Part model, mm, in its own coordinate system. A direction names the side the tool comes from. Coordinates: 2 decimals unless noted, no trailing zeros. Loops run counter-clockwise (first coordinate to the right, second up) from the corner with the lowest first, then second, coordinate; pieces in that order, holes last. Notation, with made-up numbers: (-23.5, 49.5) -> (-17.5, 49.5) arc R5 cw to (-17.5, 58.5) -> close; hole circle Ø7 at (-0.75, 52.5). An arc over 180 degrees is marked (long way). Use one line per item in the form item = value. Start each with the question number.
(1) 3-axis set-ups, long thin cutter, end or side, ignore diameter. For faces 5 (the flat face through (15.7, 2.5, -17.8)), 6 (the cylindrical face through (-14.635, 2.007, 6.999)), 7 (the cylindrical face through (11.5, 1, 6.9)): which of +Z, -Z, +X, -X, +Y, -Y reach the whole face in a straight line?
(2) Band-saw the part on B-B on x = 0. Count the separate pieces of the cut face and the enclosed holes in it, then the cut area to 3 significant figures.
(3) Band-saw the part on A-A on z = -5. Give the cut face in (x, y), then the cut area to 4 significant figures.
(4) Pin check, flat tips, straight feed: P1, Ø5, axis at x = 0, z = -5, coming from the -Y side; P2, Ø2, axis at x = 13, z = 6, coming from the +Y side; P3, Ø3, axis at y = 4.5, z = -34, coming from the +X side; P4, Ø0.5, axis at x = -13.5, y = 2, coming from the +Z side. Stop position of each tip, or through.
(5) Drill centre lines: L1, parallel to Z at x = 0, y = 0.3; L2, parallel to Z at x = -2.5, y = 0.6; L3, parallel to X at y = 0.35, z = -5. Where is each one in solid material? Low to high. Write a range as [from, to].
(6) Mould opens along X. For faces 1 (the flat face through (13, 2, 5.3)), 2 (the flat face through (11.92, 2, 6)), 3 (the cylindrical face through (-12.205, 2.007, 6.999)), 4 (the cylindrical face through (-17.08, 0.76, 12.4)) say: +X half, -X half, draft (parallel to the pull), parting line (faces both ways), or undercut.
```python
from build123d import *

# Parameters (mm, degrees)
SKETCH1_W               = 35.3
SKETCH1_H               = 26
BOSS_EXTRUDE1_DEPTH     = 1.5
SKETCH2_W               = 31.8
SKETCH2_H               = 1.5
BOSS_EXTRUDE2_DEPTH     = 3.8
CUT_EXTRUDE1_DEPTH      = 23.247752695
CUT_EXTRUDE1_DEPTH_BACK = 23.247752695
SKETCH3_R               = 2
CHAMFER1_SIZE           = 2
CHAMFER1_SIZE2          = 1
FILLET1_R               = 2
BOSS_EXTRUDE3_DEPTH     = 30
FILLET2_R               = 2
SKETCH6_W               = 3
SKETCH6_H               = 2
BOSS_EXTRUDE4_DEPTH     = 1
FILLET4_R               = 1
SKETCH7_W               = 1.743977538
SKETCH7_H               = 6.350659455
SKETCH7_W_2             = 2.282976844
SKETCH7_H_2             = 7.649157782
CUT_EXTRUDE2_DEPTH      = 37.494691395
CUT_EXTRUDE5_DEPTH      = 55.674605623
CUT_EXTRUDE5_DEPTH_BACK = 55.674605623
CUT_EXTRUDE6_DEPTH      = 47.63649323
CUT_EXTRUDE6_DEPTH_BACK = 47.63649323
CUT_EXTRUDE7_START      = -1.5
CUT_EXTRUDE7_DEPTH      = 1


with BuildPart() as part:
    # Sketch1 → Boss-Extrude1 (new body)
    with BuildSketch(Plane(origin=(0, 0, 0), x_dir=(1, 0, 0), z_dir=(0, 1, 0))):
        Rectangle(SKETCH1_W, SKETCH1_H)
    extrude(amount=BOSS_EXTRUDE1_DEPTH)

    # Sketch2 → Boss-Extrude2 (add)
    with BuildSketch(Plane(origin=(0, 1.5, 0), x_dir=(1, 0, 0), z_dir=(0, 1, 0))):
        with Locations((0, 12.25)):
            Rectangle(SKETCH2_W, SKETCH2_H)
    extrude(amount=BOSS_EXTRUDE2_DEPTH)

    # Sketch3 → Cut-Extrude1 (cut, two sides: drawn at the far end of the back side and taken through both)
    with BuildSketch(Plane(origin=(0, 1.5, 0), x_dir=(1, 0, 0), z_dir=(0, 1, 0)).offset(-CUT_EXTRUDE1_DEPTH_BACK)):
        with Locations(Location((0, 5, 0), (0, 0, 270))):
            Circle(SKETCH3_R)
    extrude(amount=CUT_EXTRUDE1_DEPTH + CUT_EXTRUDE1_DEPTH_BACK, mode=Mode.SUBTRACT)

    # Chamfer1
    chamfer1_edges = [part.edges().sort_by_distance(p)[0] for p in [
        (0, 1.5, -7),
    ]]
    chamfer1_side = [part.faces().sort_by_distance(p)[0] for p in [
        (0, 1.5, 0.754672273),
    ]]
    chamfer(chamfer1_edges, length=CHAMFER1_SIZE, length2=CHAMFER1_SIZE2, reference=chamfer1_side[0])

    # Fillet1
    fillet1_edges = [part.edges().sort_by_distance(p)[0] for p in [
        (17.65, 0.75, 13),
        (-17.65, 0.75, 13),
    ]]
    fillet(fillet1_edges, radius=FILLET1_R)

    # Sketch4 → Boss-Extrude3 (add)
    with BuildSketch(Plane(origin=(0, 0, -13), x_dir=(-1, 0, 0), z_dir=(0, 0, -1))):
        Polygon((-15.9, 5.3), (-15.9, 1.5), (-17.65, 1.5), (-17.65, 0), (17.65, 0), (17.65, 1.5), (15.9, 1.5), (15.9, 5.3), align=None)
    extrude(amount=BOSS_EXTRUDE3_DEPTH)

    # Fillet2
    fillet2_edges = [part.edges().sort_by_distance(p)[0] for p in [
        (-17.65, 0.75, -43),
        (17.65, 0.75, -43),
    ]]
    fillet(fillet2_edges, radius=FILLET2_R)

    # Sketch6 → Boss-Extrude4 (add)
    with BuildSketch(Plane(origin=(0, 1.5, 0), x_dir=(1, 0, 0), z_dir=(0, 1, 0))):
        with Locations((-13.42, -6.3)):
            Rectangle(SKETCH6_W, SKETCH6_H)
        with Locations((13.42, -6.3)):
            Rectangle(SKETCH6_W, SKETCH6_H)
    extrude(amount=BOSS_EXTRUDE4_DEPTH)

    # Fillet4
    fillet4_edges = [part.edges().sort_by_distance(p)[0] for p in [
        (-14.92, 2, 5.3),
        (14.92, 2, 5.3),
        (14.92, 2, 7.3),
        (11.92, 2, 7.3),
        (-11.92, 2, 7.3),
        (-14.92, 2, 7.3),
    ]]
    fillet(fillet4_edges, radius=FILLET4_R - 0.0001)  # a hair under: the kernel refuses the full size

    # Sketch7 → Cut-Extrude2 (cut, through all)
    with BuildSketch(Plane.XY.offset(-11.5)):
        with Locations((-16.571988769, 4.675329728)):
            Rectangle(SKETCH7_W, SKETCH7_H)
        with Locations((16.841488422, 5.324578891)):
            Rectangle(SKETCH7_W_2, SKETCH7_H_2)
    extrude(amount=-CUT_EXTRUDE2_DEPTH, mode=Mode.SUBTRACT)

    # Sketch10 → Cut-Extrude5 (cut, two sides: drawn at the far end of the back side and taken through both)
    with BuildSketch(Plane(origin=(15.7, 0, 0), x_dir=(0, 0, -1), z_dir=(1, 0, 0)).offset(-CUT_EXTRUDE5_DEPTH_BACK)):
        with BuildLine():
            Line((12.925241615, 5.3), (13.354629123, 9.309511059))
            Line((13.354629123, 9.309511059), (48.378706372, 9.920156593))
            Line((48.378706372, 9.920156593), (42.999374902, 1.5))
            add(Edge.make_bspline(
                [(12.925241615, 5.3), (21.883759375, -0.11684658), (33.318611191, 2.283464976), (42.999374902, 1.5)],
                knots=[0, 0, 0, 0, 1, 1, 1, 1], degree=3))
        make_face()
    extrude(amount=CUT_EXTRUDE5_DEPTH + CUT_EXTRUDE5_DEPTH_BACK, mode=Mode.SUBTRACT)

    # Sketch12 → Cut-Extrude6 (cut, two sides: drawn at the far end of the back side and taken through both)
    with BuildSketch(Plane(origin=(0, 1.5, 0), x_dir=(1, 0, 0), z_dir=(0, 1, 0)).offset(-CUT_EXTRUDE6_DEPTH_BACK)):
        with BuildLine():
            Line((-2.9, -5), (2.9, -5))
            ThreePointArc((2.9, -5), (4.75, -6.85), (2.9, -8.7))
            Line((2.9, -8.7), (-2.9, -8.7))
            ThreePointArc((-2.9, -8.7), (-4.75, -6.85), (-2.9, -5))
        make_face()
    extrude(amount=CUT_EXTRUDE6_DEPTH + CUT_EXTRUDE6_DEPTH_BACK, mode=Mode.SUBTRACT)

    # Sketch13 → Cut-Extrude7 (cut)
    with BuildSketch(Plane.XZ.offset(CUT_EXTRUDE7_START)):
        with BuildLine():
            Line((-8, 10.35), (8, 10.35))
            ThreePointArc((8, 10.35), (11.5, 6.85), (8, 3.35))
            Line((8, 3.35), (-8, 3.35))
            ThreePointArc((-8, 3.35), (-11.5, 6.85), (-8, 10.35))
        make_face()
    extrude(amount=CUT_EXTRUDE7_DEPTH, mode=Mode.SUBTRACT)


solid = part.part
```
A:
q1.face_5 = +Z, -Z, +X, +Y
q1.face_6 = +Z, -X, +Y
q1.face_7 = +Y
q2.separate_pieces = 3
q2.enclosed_holes = 0
q2.area = 93.9 mm²
q3.outline = (-17.65, 0) -> (-2, 0) -> (-2, 0.5) -> (-4, 1.5) -> (-17.65, 1.5) -> close; (2, 0) -> (17.65, 0) -> (17.65, 1.5) -> (4, 1.5) -> (2, 0.5) -> close
q3.area = 44.95 mm²
q4.P1 = 0
q4.P2 = 2.5
q4.P3 = through
q4.P4 = 7.3
q5.L1 = [-43, -7], [-3, 5], [8.7, 13]
q5.L2 = [-43, 3.35], [10.35, 13]
q5.L3 = [-17.65, -2], [2, 17.65]
q6.face_1 = draft
q6.face_2 = undercut
q6.face_3 = undercut
q6.face_4 = -X half
